Drawing for the job (mm, zero at the part's lowest x, y, z). A direction names the side the tool comes from. Coordinates: 2 decimals unless noted, no trailing zeros. Write each loop counter-clockwise with the first axis right and the second up, starting at its lowest first coordinate (ties: lowest second). Pieces come first, ordered by that corner, then holes. Notation, with made-up numbers: M 76,-36.5 L 126,-36.5 A28 ccw 126,1.5 Z; hole C 8,24 d5. An arc over 180 degrees is marked long. Use a Markdown table: item, result. Add a question column.
Q1. Tool access for the marked faces 4, 5 and 6: list every direction of +Z, -Z, +X, -X, +Y, -Y with a clear straight run to the whole face (end or side of a thin tool).
Q2. Wall check: L1, parallel to Z at x = 9.5, y = 9; L2, parallel to Y at x = 6.5, z = 43; L3, parallel to Y at x = 32, z = 47.5. Give the ranges that are in metal, low to high. Write a range as from..to.
Q3. Pin check, flat tips, straight feed: pin 1 Ø8 at (x, y) = (23, 45) entering from -Z; pin 2 Ø7.5 at (x, z) = (19, 44) entering from +Y; pin 3 Ø8 at (y, z) = (23, 73) entering from -X; pin 4 Ø1 at (x, y) = (38.5, 20) entering from +Z. Stop position of each tip, or through.
Q4. Slice it at A-A on y = 8.5. Write the cut outline in (x, z), then the cut area to 3 significant figures.
Q5. Slice it at C-C on x = 25. Write the cut outline in (y, z), then the cut area to 4 significant figures.
Q6. Slice it at D-D on y = 26. Write the cut outline in (x, z), then the cut area to 3 significant figures.
Q7. Slice it at B-B on z = 45. Write the cut outline in (x, y), then the cut area to 3 significant figures.
Q8. Mould opens along Z. For the marked faces 1, 2 and 3 say: released by +Z, released by -Z, zero draft, split by the parting line, or undercut.
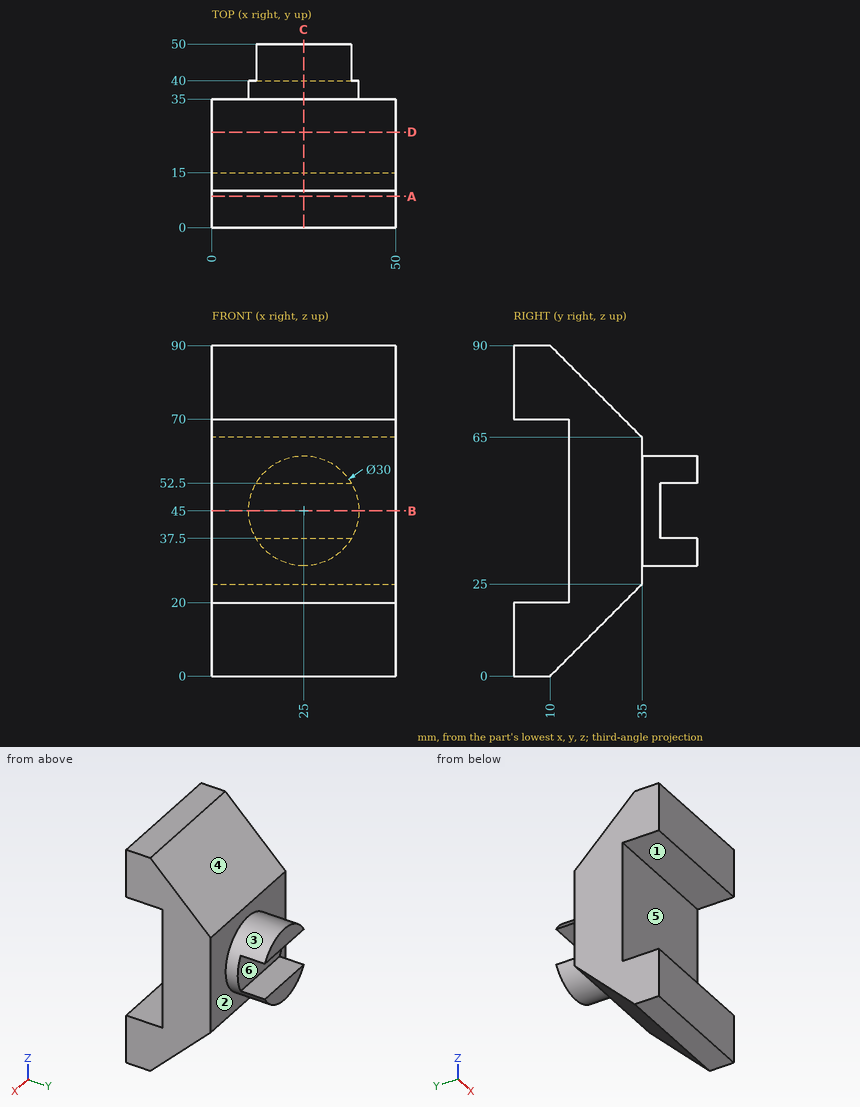
Recorded:
| question | item | result |
|---|---|---|
| 1 | face 4 | +Z, +X, -X, +Y |
| 1 | face 5 | +X, -X, -Y |
| 1 | face 6 | +X, -X, +Y |
| 2 | L1 | 0..20, 70..90 |
| 2 | L2 | 15..35 |
| 2 | L3 | 15..40 |
| 3 | pin 1 | z = 30 |
| 3 | pin 2 | y = 40 |
| 3 | pin 3 | x = 0 |
| 3 | pin 4 | z = 80.5 |
| 4 | outline | M 0,0 L 50,0 L 50,20 L 0,20 Z; M 0,70 L 50,70 L 50,90 L 0,90 Z |
| 4 | area | 2,000 mm² |
| 5 | outline | M 0,0 L 10,0 L 35,25 L 35,30 L 50,30 L 50,37.5 L 40,37.5 L 40,52.5 L 50,52.5 L 50,60 L 35,60 L 35,65 L 10,90 L 0,90 L 0,70 L 15,70 L 15,20 L 0,20 Z |
| 5 | area | 2,075 mm² |
| 6 | outline | M 0,16 L 50,16 L 50,74 L 0,74 Z |
| 6 | area | 2,900 mm² |
| 7 | outline | M 0,15 L 50,15 L 50,35 L 40,35 L 40,40 L 10,40 L 10,35 L 0,35 Z |
| 7 | area | 1,150 mm² |
| 8 | face 1 | undercut |
| 8 | face 2 | zero draft |
| 8 | face 3 | split by the parting line |
